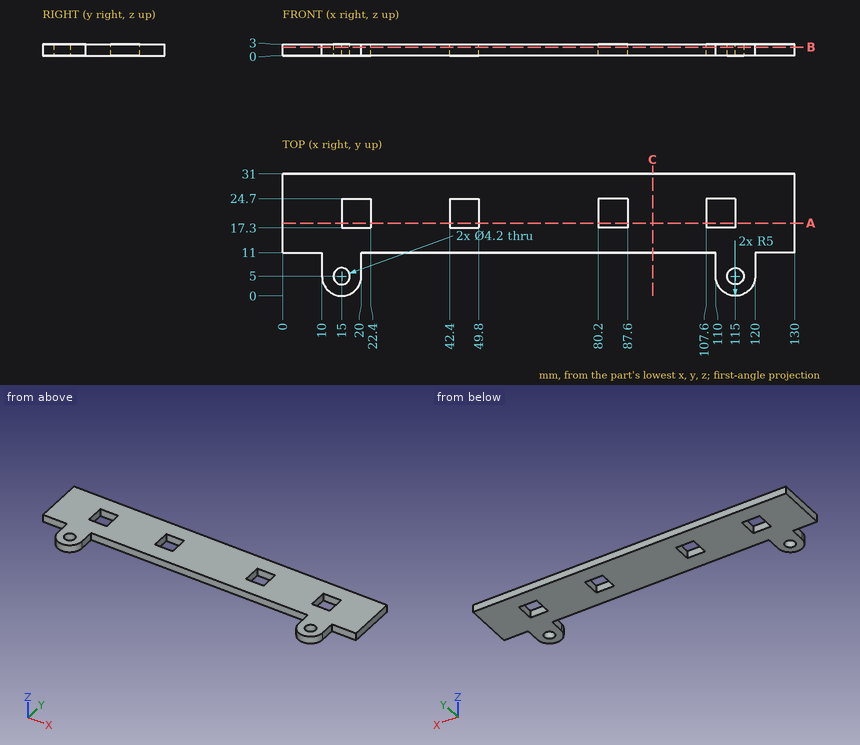
Could you check a few things on this drawing? It's one solid part, dimensions in mm from its lowest x, y, z. Give positions to 0.01 mm unless a question says otherwise; leave off trailing zeros. Write each loop counter-clockwise with the first axis right and the second up, starting at its lowest first coordinate (ties: lowest second). Pieces come first, ordered by that corner, then holes. Notation, with made-up numbers: (-15, -34) -> (4, -34) arc R33 ccw to (4, 1) -> close; hole circle Ø10 at (71.25, -32). An arc over 180 degrees is marked (long way). Answer as CSV lines item,"result". Start each with the question number.
(1) Please list where these lines run through material, in increasing order: line 1 (X direction, y = 23, z = 0.3); line 2 (Y direction, x = 43, z = 2.35); line 3 (Y direction, x = 16, z = 1.45).
(2) If we section it at A-A, the plane y = 18.5: Write out the boundary of the cut face in (x, z), and give its area (3 significant figures).
(3) If we section it at C-C, the plane x = 94: Write out the boundary of the cut face in (y, z), and give its area (3 significant figures).
(4) I'm going to push flat-ended pins straight in: pin 1 Ø0.9 at (x, z) = (46.5, 2) entering from -Y; pin 2 Ø1.5 at (y, z) = (8, 2) entering from -X. Where does each tip first touch, or does it pass through?
(5) If we section it at B-B, the plane z = 2.2: Give the number of separate pieces and of enclosed holes in the cut face, and give its area (3 significant figures).
Answer list:
1,line 1,"0 to 15, 22.4 to 42.4, 49.8 to 80.2, 87.6 to 107.6, 115 to 130"
1,line 2,"11 to 17.3, 24.7 to 31"
1,line 3,"0.1 to 3.15, 6.85 to 17.3, 24.7 to 31"
2,outline,"(0, 0) -> (15, 0) -> (15, 3) -> (0, 3) -> close; (22.4, 0) -> (42.4, 0) -> (42.4, 3) -> (22.4, 3) -> close; (49.8, 0) -> (80.2, 0) -> (80.2, 3) -> (49.8, 3) -> close; (87.6, 0) -> (107.6, 0) -> (107.6, 3) -> (87.6, 3) -> close; (115, 0) -> (130, 0) -> (130, 3) -> (115, 3) -> close"
2,area,"301 mm^2"
3,outline,"(11, 0) -> (31, 0) -> (31, 3) -> (11, 3) -> close"
3,area,"60.0 mm^2"
4,pin 1,"y = 11"
4,pin 2,"x = 10"
5,separate pieces,"1"
5,enclosed holes,"6"
5,area,"2,550 mm^2"
